CAD build for the part. Positions are in the model's coordinates, mm. Round coordinates to 2 decimals unless told otherwise and drop trailing zeros. Order: outer loops, then holes, each group sorted by start corner. A loop starts at its lowest first (then second) coordinate and runs counter-clockwise, first axis right, second up. Notation, with made-up numbers: (33.5, 47) -> (47.5, 47) arc R7 ccw to (47.5, 59) -> close; hole circle Ø5 at (75.5, 89.5). An arc over 180 degrees is marked (long way). Answer as CSV lines item,"result". Start each with the question number.
from build123d import *

# Parameters (mm, degrees)
GUARD_BASE_R     = 30
GUARD_DEPTH      = 5
AXLE_HOLE_BASE_R = 19.25
AXLE_HOLE_DEPTH  = 6


with BuildPart() as part:
    # Guard base → Guard (new body)
    with BuildSketch(Plane.XY):
        Circle(GUARD_BASE_R)
    extrude(amount=GUARD_DEPTH)

    # Axle hole base → Axle hole (cut, through all)
    with BuildSketch(Plane.XY.offset(5)):
        Circle(AXLE_HOLE_BASE_R)
    extrude(amount=-AXLE_HOLE_DEPTH, mode=Mode.SUBTRACT)

    # Mate ring room base → Mate ring room (revolve, cut)
    with BuildSketch(Plane(origin=(0, 0, 0), x_dir=(1, 0, 0), z_dir=(0, 1, 0))):
        Polygon((19.25, -5), (20, -5), (19.25, -4.25), align=None)
        Polygon((19.25, 0), (20, 0), (19.25, -0.75), align=None)
    revolve(axis=Axis((0, 0, 0), (0, 0, -1)), mode=Mode.SUBTRACT)


solid = part.part
Item 1: Pin check, flat tips, straight feed: pin 1 (10 mm diameter, centred on x = -1, y = 18.5, fed in from -Z); pin 2 (3 mm diameter, centred on y = 9, z = 2, fed in from -X); pin 3 (1.5 mm diameter, centred on x = -5, z = 1.5, fed in from +Y). Stop position of each tip, or through.
Item 2: Band-saw the part on A-A, the plane x = 0. Give the cut face in (y, z).
Item 3: Mould opens along X. For faces 1 (the cylindrical face through (-15.28, -11.71, 2.52)), 2 (the cylindrical face through (-29.97, 1.32, 2.46)), 3 (the flat face through (6, -20, 0)) say: released by +X, released by -X, zero draft, split by the parting line, or undercut.
Item 4: Band-saw the part on C-C, the plane x = -22.5. Give the cut face in (y, z).
Item 5: Probe line 1 (Y direction, x = 0, z = 1.9); line 2 (X direction, y = 14, z = 3.5); line 3 (Y direction, x = -11, z = 0.6). List the from-to ranges inside material, lowest first.
Values:
1,pin 1,"z = 0"
1,pin 2,"x = -29.05"
1,pin 3,"y = 29.7"
2,outline,"(-30, 0) -> (-20, 0) -> (-19.25, 0.75) -> (-19.25, 4.25) -> (-20, 5) -> (-30, 5) -> close; (19.25, 0.75) -> (20, 0) -> (30, 0) -> (30, 5) -> (20, 5) -> (19.25, 4.25) -> close"
3,face 1,"undercut"
3,face 2,"split by the parting line"
3,face 3,"zero draft"
4,outline,"(-19.84, 0) -> (19.84, 0) -> (19.84, 5) -> (-19.84, 5) -> close"
5,line 1,"-30 to -19.25, 19.25 to 30"
5,line 2,"-26.53 to -13.21, 13.21 to 26.53"
5,line 3,"-27.91 to -15.98, 15.98 to 27.91"
